Geometry check sheet. Reference: drawing and pictorial views, mm from the part's lowest x, y, z. A direction names the side the tool comes from. Give positions to 0.01 mm unless a question says otherwise; leave off trailing zeros. Order: outer loops, then holes, each group sorted by start corner. A loop starts at its lowest first (then second) coordinate and runs counter-clockwise, first axis right, second up. Notation, with made-up numbers: (57.25, -7) -> (75.25, -7) arc R30 ccw to (75.25, 16) -> close; hole circle Ø3 at (-20.5, 75). An arc over 180 degrees is marked (long way). Write each question's results on one line, items separated by ' | '. Start each with the question number.
1. Set-up check for the marked faces 1 and 2: record each of +Z, -Z, +X, -X, +Y, -Y from which the full face is reachable in a straight line by a thin tool's end or side.
2. Cross-section at B-B, the plane y = 140.5. Enter the section's corners in (x, z), then the cut area to 3 significant figures.
3. Depth check by flat-ended pin: pin 1 Ø2 at (y, z) = (129.5, 42) entering from -X; pin 2 Ø2 at (y, z) = (55, 48.5) entering from +X; pin 3 Ø6 at (x, y) = (18.5, 120.5) entering from +Z; pin 4 Ø3 at (x, y) = (13, 132.5) entering from -Z. Enter the tip coordinate at first touch or a pass-through.
4. Cross-section at A-A, the plane x = 50. Enter the section's corners in (y, z), then the cut area to 3 significant figures.
5. Cross-section at C-C, the plane y = 24. Enter the section's corners in (x, z), then the cut area to 3 significant figures.
6. Material ranges on L1, parallel to Y at x = 34, z = 44; L2, parallel to X at y = 124.5, z = 49.5; L3, parallel to Y at x = 79, z = 13.5, recorded low to high. Write a range as from..to.
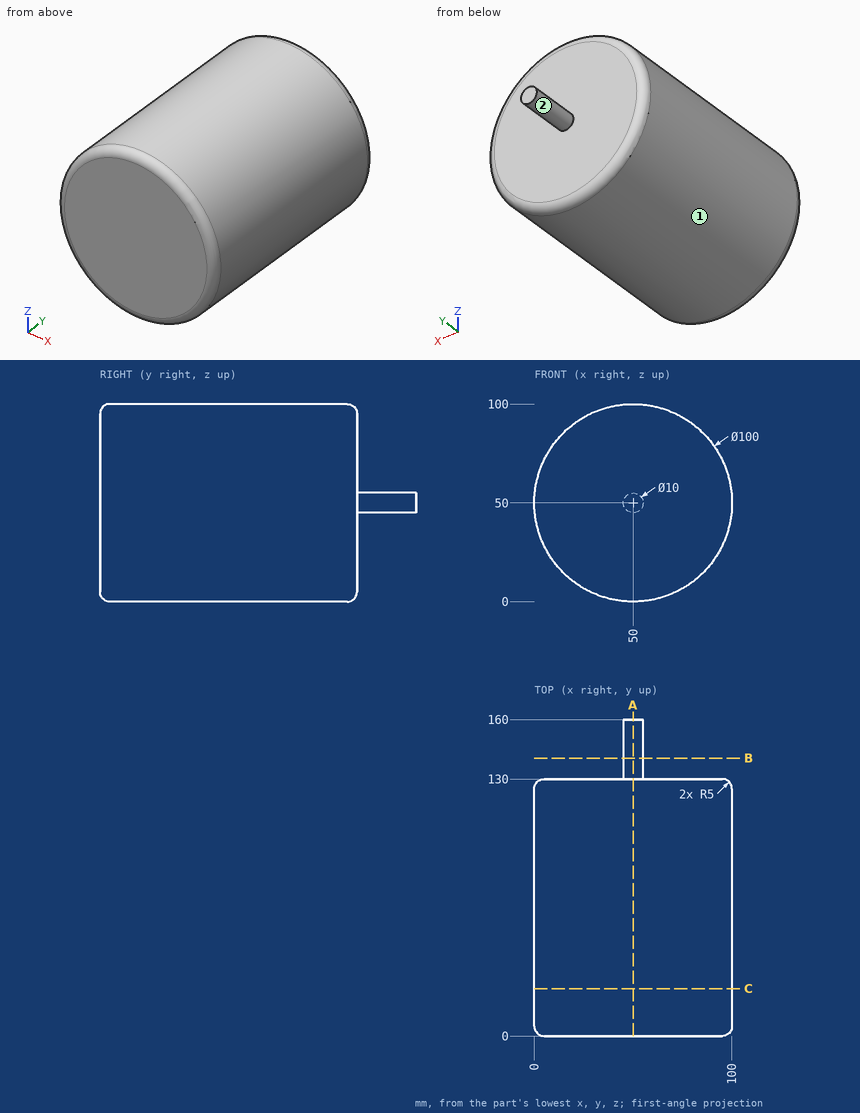
Results below:
1) face 1: +Y, -Y | face 2: +Y
2) outline: circle Ø10 at (50, 50) | area: 78.5 mm²
3) pin 1: stops at x = 2.08 | pin 2: stops at x = 100 | pin 3: stops at z = 91.08 | pin 4: passes through
4) outline: (0, 5) arc R5 ccw to (5, 0) -> (125, 0) arc R5 ccw to (130, 5) -> (130, 45) -> (160, 45) -> (160, 55) -> (130, 55) -> (130, 95) arc R5 ccw to (125, 100) -> (5, 100) arc R5 ccw to (0, 95) -> close | area: 13,300 mm²
5) outline: circle Ø100 at (50, 50) | area: 7,850 mm²
6) L1: y = 0..130 | L2: x = 0..100 | L3: y = 0.27..129.73
